Build history of the part. All positions in model axes, mm. A direction names the side the tool comes from. Coordinates: 2 decimals unless noted, no trailing zeros. Order: outer loops, then holes, each group sorted by start corner. A loop starts at its lowest first (then second) coordinate and runs counter-clockwise, first axis right, second up. Notation, with made-up numbers: (49, 47) - (95, 47) arc R25 ccw to (95, 66) - close; hole circle Ø11 at (42.5, 30.25). An arc over 180 degrees is marked (long way). Return JSON: item names as keys, results as strings.
from build123d import *

# Parameters (mm, degrees)
SKETCH_1_W          = 141
SKETCH_1_H          = 50
EXTRUDE_1_DEPTH     = 1.6
SKETCH_2_R          = 1.75
CUT_EXTRUDE_1_DEPTH = 10
SKETCH_3_R          = 1.75
CUT_EXTRUDE_2_DEPTH = 10
SKETCH_4_R          = 1.234132003
EXTRUDE_2_DEPTH     = 5
SKETCH_7_W          = 122
SKETCH_7_H          = 10
EXTRUDE_3_DEPTH     = 11
SKETCH_8_W          = 127
SKETCH_8_H          = 11
EXTRUDE_4_DEPTH     = 2
SKETCH_6_R          = 0.888976415
EXTRUDE_5_DEPTH     = 5
SKETCH_9_W          = 6.5
SKETCH_9_H          = 10
CUT_EXTRUDE_3_DEPTH = 11


with BuildPart() as part:
    # 草图1 → 凸台-拉伸1 (new body)
    with BuildSketch(Plane(origin=(0, 0, 0), x_dir=(1, 0, 0), z_dir=(0, 1, 0))):
        Rectangle(SKETCH_1_W, SKETCH_1_H)
    extrude(amount=EXTRUDE_1_DEPTH)

    # 草图2 → 切除-拉伸1 (cut)
    with BuildSketch(Plane(origin=(0, 1.6, 0), x_dir=(1, 0, 0), z_dir=(0, 1, 0))):
        with Locations((-67.5, -22.25)):
            Circle(SKETCH_2_R)
        with Locations((-67.5, 20.75)):
            Circle(SKETCH_2_R)
        with Locations((67.5, 20.75)):
            Circle(SKETCH_2_R)
        with Locations((67.5, -22.25)):
            Circle(SKETCH_2_R)
    extrude(amount=-CUT_EXTRUDE_1_DEPTH, mode=Mode.SUBTRACT)

    # 草图3 → 切除-拉伸2 (cut)
    with BuildSketch(Plane(origin=(0, 1.6, 0), x_dir=(1, 0, 0), z_dir=(0, 1, 0))):
        with Locations((-63.5, 20)):
            Circle(SKETCH_3_R)
        with Locations((-24, 20)):
            Circle(SKETCH_3_R)
        with Locations((-63.5, -3)):
            Circle(SKETCH_3_R)
        with Locations((-24, -3)):
            Circle(SKETCH_3_R)
        with Locations((15.25, -3)):
            Circle(SKETCH_3_R)
        with Locations((57.75, -3)):
            Circle(SKETCH_3_R)
        with Locations((15.25, 20)):
            Circle(SKETCH_3_R)
        with Locations((57.75, 20)):
            Circle(SKETCH_3_R)
    extrude(amount=-CUT_EXTRUDE_2_DEPTH, mode=Mode.SUBTRACT)

    # 草图4 → 凸台-拉伸2 (add)
    with BuildSketch(Plane(origin=(0, 0, 0), x_dir=(1, 0, 0), z_dir=(0, 1, 0))):
        with Locations((-47.078898204, 20)):
            Circle(SKETCH_4_R)
        with Locations((-43.75, 20)):
            Circle(SKETCH_4_R)
        with Locations((-40.421101796, 20)):
            Circle(SKETCH_4_R)
    extrude(amount=-EXTRUDE_2_DEPTH)

    # 草图7 → 凸台-拉伸3 (add)
    with BuildSketch(Plane.XZ):
        with Locations((-7.5, -6.5)):
            Rectangle(SKETCH_7_W, SKETCH_7_H)
    extrude(amount=EXTRUDE_3_DEPTH)

    # 草图8 → 凸台-拉伸4 (add)
    with BuildSketch(Plane(origin=(0, 1.6, 0), x_dir=(1, 0, 0), z_dir=(0, 1, 0))):
        with Locations((-6, 9.5)):
            Rectangle(SKETCH_8_W, SKETCH_8_H)
    extrude(amount=EXTRUDE_4_DEPTH)

    # 草图6 → 凸台-拉伸5 (add)
    with BuildSketch(Plane(origin=(0, 0, 0), x_dir=(1, 0, 0), z_dir=(0, 1, 0))):
        with Locations((67.875178123, 10.882897677)):
            Circle(SKETCH_6_R)
        with Locations((67.875178123, 6.093097389)):
            Circle(SKETCH_6_R)
    extrude(amount=-EXTRUDE_5_DEPTH)

    # 草图9 → 切除-拉伸3 (cut)
    with BuildSketch(Plane.XZ.offset(11)):
        with Locations((-55.25, -6.5)):
            Rectangle(SKETCH_9_W, SKETCH_9_H)
    extrude(amount=-CUT_EXTRUDE_3_DEPTH, mode=Mode.SUBTRACT)


solid = part.part
1. Cut at B-B on x = -63.5. Give the cut face in (y, z).
Check values:
{"outline": "(-11, -11.5) - (0, -11.5) - (0, -18.25) - (1.6, -18.25) - (1.6, -15) - (3.6, -15) - (3.6, -4) - (1.6, -4) - (1.6, 1.25) - (0, 1.25) - (0, -1.5) - (-11, -1.5) - close; (0, -25) - (1.6, -25) - (1.6, -21.75) - (0, -21.75) - close; (0, 4.75) - (1.6, 4.75) - (1.6, 25) - (0, 25) - close"}
2. Mould opens along Z. For faces 6 (the cylindrical face through (16.867, 0.811, 3.67)), 7 (the flat face through (-58.5, -6, -7)), 8 (the flat face through (0, -5, -1.5)) say: pulls with the +Z half, pulls with the -Z half, needs draft (parallel to the pull), parting line crosses it, or undercut.
Check values:
{"face 6": "undercut", "face 7": "needs draft", "face 8": "pulls with the +Z half"}
3. Cut at C-C on x = -43.75. Give the cut face in (y, z), plus the area to 3 significant figures.
Check values:
{"outline": "(-11, -11.5) - (0, -11.5) - (0, -18.77) - (-5, -18.77) - (-5, -21.23) - (0, -21.23) - (0, -25) - (1.6, -25) - (1.6, -15) - (3.6, -15) - (3.6, -4) - (1.6, -4) - (1.6, 25) - (0, 25) - (0, -1.5) - (-11, -1.5) - close", "area": "224 mm²"}
4. Cut at A-A on y = -9.5. Give the cut face in (x, z).
Check values:
{"outline": "(-68.5, -11.5) - (-58.5, -11.5) - (-58.5, -1.5) - (-68.5, -1.5) - close; (-52, -11.5) - (53.5, -11.5) - (53.5, -1.5) - (-52, -1.5) - close"}
5. Drop flat-ended pins along their axis: pin 1 (3 mm diameter, centred on x = 36.5, y = -5.5, fed in from +Z); pin 2 (2 mm diameter, centred on x = 19.5, z = 8.5, fed in from -Y); pin 3 (1.6 mm diameter, centred on y = 2.5, z = -8.5, fed in from +X); pin 4 (12 mm diameter, centred on x = 22, z = -1, fed in from +Y). Give the stop position or say it passes through.
Check values:
{"pin 1": "z = -1.5", "pin 2": "y = 0", "pin 3": "x = 57.5", "pin 4": "y = 3.6"}
6. Tool access for faces 1 (the flat face through (-44, -5, -20)), 2 (the cylindrical face through (-61.883, 0.811, 3.67)), 3 (the flat face through (-64, -5, -11.5)), 4 (the cylindrical face through (-48.06, -2.46, -19.25)), 5 (the flat face through (-68.5, -5, -7)): list every direction of +Z, -Z, +X, -X, +Y, -Y with a clear straight run to the whole face (end or side of a thin tool).
Check values:
{"face 1": "-Z, +X, -X, -Y", "face 2": "+Y, -Y", "face 3": "-Z, -X, -Y", "face 4": "-Y", "face 5": "+Z, -Z, -X, -Y"}
7. Probe L1, parallel to Z at x = -67.5, y = 0.4; L2, parallel to Z at x = 15.25, y = 1.2; L3, parallel to X at y = 0.5, z = 22.25. List the from-to ranges inside material, lowest first.
Check values:
{"L1": "-25 to -22.5, -19 to 20.5, 24 to 25", "L2": "-25 to -21.75, -18.25 to 1.25, 4.75 to 25", "L3": "-70.5 to -69.25, -65.75 to 65.75, 69.25 to 70.5"}
8. Cut at D-D on y = -2.5. Give the cut face in (x, z).
Check values:
{"outline": "(-68.5, -11.5) - (-58.5, -11.5) - (-58.5, -1.5) - (-68.5, -1.5) - close; (-52, -11.5) - (53.5, -11.5) - (53.5, -1.5) - (-52, -1.5) - close; circle Ø2.47 at (-47.08, -20); circle Ø2.47 at (-43.75, -20); circle Ø2.47 at (-40.42, -20); circle Ø1.78 at (67.88, -10.88); circle Ø1.78 at (67.88, -6.09)"}
